Design review of the part shown in the three views and the two pictorial views. Dimensions are in mm from the part's minimum x, y and z. A direction names the side the tool comes from. Coordinates: 2 decimals unless noted, no trailing zeros. Write each loop counter-clockwise with the first axis right and the second up, starting at its lowest first coordinate (ties: lowest second). Pieces come first, ordered by that corner, then holes. Notation, with made-up numbers: (55, -26.5) - (89, -26.5) arc R18 cw to (89, -15.5) - close; hole circle Ø6 at (69.5, -6). An arc over 180 degrees is marked (long way). Write each question's results on one line, items separated by ' | '.
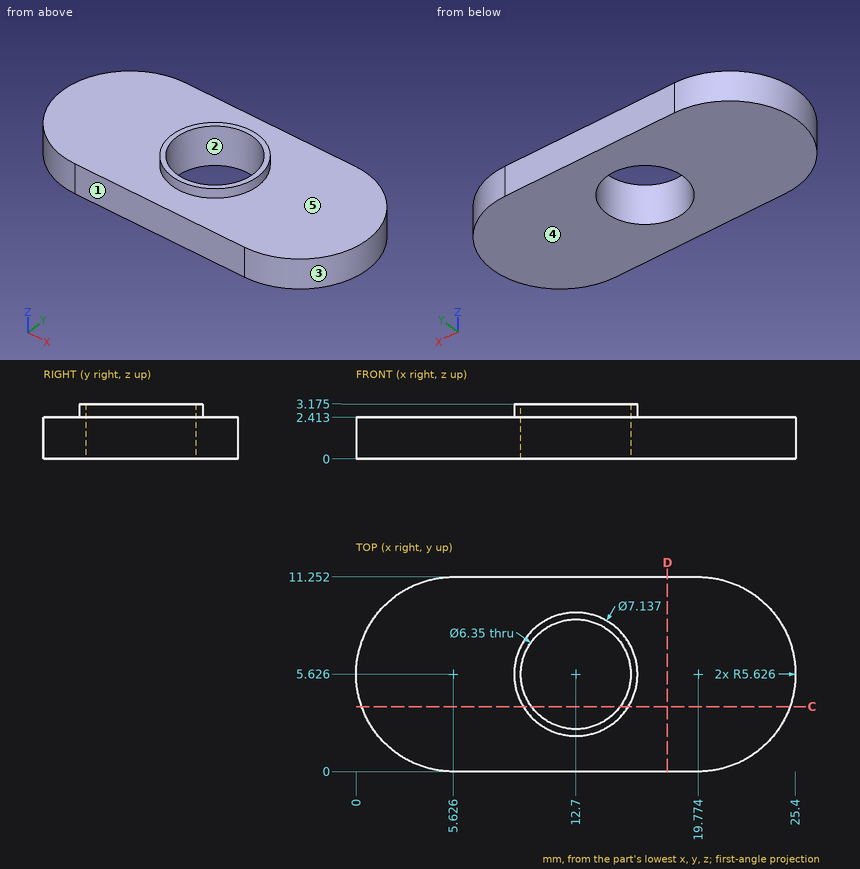
Q1. Take a section at C-C on y = 3.75. State the section outline as (x, z) points (1 decimal), plus the area to 3 significant figures.
Results found:
outline: (0.3, 0) - (10.1, 0) - (10.1, 3.2) - (9.7, 3.2) - (9.7, 2.4) - (0.3, 2.4) - close; (15.3, 0) - (25.1, 0) - (25.1, 2.4) - (15.7, 2.4) - (15.7, 3.2) - (15.3, 3.2) - close | area: 48.1 mm2
Q2. Mouldability with a two-part tool opening along X and no side actions: class the marked faces 1, 2 and 3 as pulls with the +X half, pulls with the -X half, needs draft (parallel to the pull), parting line crosses it, or undercut.
Results found:
face 1: needs draft | face 2: undercut | face 3: pulls with the +X half
Q3. Take a section at D-D on x = 18. State the section outline as (y, z) points.
Results found:
outline: (0, 0) - (11.25, 0) - (11.25, 2.41) - (0, 2.41) - close
Q4. For pin 1 (1.5 mm diameter, centred on y = 1.5, z = 1.5, fed in from +X) (1 decimal); pin 2 (1 mm diameter, centred on x = 8.5, y = 3.5, fed in from +Z), all flat-tipped, find the tip position at first contact; note any pin that passes through.
Results found:
pin 1: x = 24.3 | pin 2: z = 2.41
Q5. Wall thickness on line 1 along Y through (x, z) = (12.7, 2.2); line 2 along X through (y, z) = (5.75, 2.75); line 3 along X through (y, z) = (5.75, 1.3): over which ranges is each line inside the solid? List them lowest first. Write a range as from..to.
Results found:
line 1: 0..2.45, 8.8..11.25 | line 2: 9.13..9.53, 15.87..16.27 | line 3: 0..9.53, 15.87..25.4
Q6. For the marked faces 4 and 5, list the 3-axis set-ups (+Z, -Z, +X, -X, +Y, -Y) from which the entire face can be reached by the end or side of a thin tool; tool diameter is ignored.
Results found:
face 4: -Z, +X, -X, +Y, -Y | face 5: +Z
